Read the model definition and answer for the solid it produces. Units are mm, in the model's axes. A direction names the side the tool comes from. Coordinates: 2 decimals unless noted, no trailing zeros. Order: outer loops, then holes, each group sorted by start corner. A loop starts at its lowest first (then second) coordinate and runs counter-clockwise, first axis right, second up. Notation, with made-up numbers: (-2, 55) - (2, 55) arc R38 ccw to (2, 93) - close; hole circle Ø3 at (87, 69.5). An arc over 180 degrees is marked (long way). Answer as a JSON object with one key per item and string values. Group by question number.
from build123d import *

# Parameters (mm, degrees)
BOSS_EXTRUDE1_DEPTH = 2
BOSS_EXTRUDE2_DEPTH = 2
SKETCH3_R           = 1.2
CUT_EXTRUDE1_DEPTH  = 5
SKETCH4_W           = 6
SKETCH4_H           = 6
CUT_EXTRUDE2_DEPTH  = 5


with BuildPart() as part:
    # Sketch1 → Boss-Extrude1 (new body)
    with BuildSketch(Plane(origin=(0, 0, 0), x_dir=(1, 0, 0), z_dir=(0, 1, 0))):
        with BuildLine():
            Line((-6.5, 2), (6.5, 2))
            ThreePointArc((6.5, 2), (8.5, 0), (6.5, -2))
            Line((6.5, -2), (-6.5, -2))
            ThreePointArc((-6.5, -2), (-8.5, 0), (-6.5, 2))
        make_face()
    extrude(amount=BOSS_EXTRUDE1_DEPTH)

    # Sketch2 → Boss-Extrude2 (add)
    with BuildSketch(Plane.XZ):
        with BuildLine():
            Line((-6.5, 1.15), (6.5, 1.15))
            ThreePointArc((6.5, 1.15), (7.65, 0), (6.5, -1.15))
            Line((6.5, -1.15), (-6.5, -1.15))
            ThreePointArc((-6.5, -1.15), (-7.65, 0), (-6.5, 1.15))
        make_face()
    extrude(amount=BOSS_EXTRUDE2_DEPTH)

    # Sketch3 → Cut-Extrude1 (cut, through all)
    with BuildSketch(Plane.XZ.offset(2)):
        Circle(SKETCH3_R)
    extrude(amount=-CUT_EXTRUDE1_DEPTH, mode=Mode.SUBTRACT)

    # Sketch4 → Cut-Extrude2 (cut, through all)
    with BuildSketch(Plane.XZ.offset(2)):
        with Locations((-7.5, 0)):
            Rectangle(SKETCH4_W, SKETCH4_H)
    extrude(amount=-CUT_EXTRUDE2_DEPTH, mode=Mode.SUBTRACT)


solid = part.part
1. A cutting plane is placed at A-A on x = 0. Write down the section's boundary in (y, z), and give its area (3 significant figures).
2. Given pin 1 (1.6 mm diameter, centred on x = -3.5, y = -1, fed in from +Z); pin 2 (1.6 mm diameter, centred on x = 2, y = -1, fed in from -Z); pin 3 (0.6 mm diameter, centred on x = 3, y = -0.5, fed in from +Z), each flat-ended and moving along its own axis, determine where each tip first touches the part or whether it passes through.
3. A cutting plane is placed at B-B on z = 0. Write down the section's boundary in (x, y), and give its area (3 significant figures).
4. A cutting plane is placed at C-C on y = -0.15. Write down the section's boundary in (x, z), and give its area (3 significant figures).
5. For faces 1 (the flat face through (2.1, 0, -1.4)), 2 (the flat face through (3, -1, 1.15)), 3 (the flat face through (3, -1, -1.15)), 4 (the flat face through (1, 1, 2)), 5 (the flat face through (-3, -2, 0)), determine the directions among +Z, -Z, +X, -X, +Y, -Y from which every point of the face is accessible in a straight line to the end or side of a thin tool.
6. For a pull along X with two mould halves and no side action, classify faces 6 (the cylindrical face through (1.145, -0.028, 0.36)), 7 (the flat face through (1, 1, -2)), 8 (the cylindrical face through (8.5, 1, 0)), 9 (the flat face through (-4.5, 0, 0)) as pulls with the +X half, pulls with the -X half, needs draft (parallel to the pull), parting line crosses it, or undercut.
7. Straight lines are drawn through the part: L1, parallel to X at y = 0.1, z = 0; L2, parallel to X at y = -0.9, z = 0; L3, parallel to Z at x = 0, y = 0.2. For each, find the intervals that lie inside material, in ascending order.
8. A cutting plane is placed at D-D on x = 3.75. Write down the section's boundary in (y, z), and give its area (3 significant figures).
Derived:
{
 "1": {"outline": "(0, -2) - (2, -2) - (2, -1.2) - (0, -1.2) - close; (0, 1.2) - (2, 1.2) - (2, 2) - (0, 2) - close", "area": "3.20 mm2"},
 "2": {"pin 1": "stops at z = 1.15", "pin 2": "stops at z = -1.15", "pin 3": "stops at z = 1.15"},
 "3": {"outline": "(-4.5, -2) - (-1.2, -2) - (-1.2, 2) - (-4.5, 2) - close; (1.2, -2) - (7.65, -2) - (7.65, 0) - (8.5, 0) - (8.5, 2) - (1.2, 2) - close", "area": "40.7 mm2"},
 "4": {"outline": "(-4.5, -1.15) - (-0.34, -1.15) arc R1.2 cw to (-0.34, 1.15) - (-4.5, 1.15) - close; (0.34, -1.15) - (6.5, -1.15) arc R1.15 ccw to (6.5, 1.15) - (0.34, 1.15) arc R1.2 cw to start", "area": "22.9 mm2"},
 "5": {"face 1": "+X, -Y", "face 2": "+Z, +X, -X, -Y", "face 3": "-Z, +X, -X, -Y", "face 4": "+Z, +X, -X, +Y, -Y", "face 5": "+Z, -Z, +X, -X, -Y"},
 "6": {"face 6": "undercut", "face 7": "needs draft", "face 8": "pulls with the +X half", "face 9": "pulls with the -X half"},
 "7": {"L1": "x = -4.5 to -1.2, 1.2 to 8.5", "L2": "x = -4.5 to -1.2, 1.2 to 7.65", "L3": "z = -2 to -1.2, 1.2 to 2"},
 "8": {"outline": "(-2, -1.15) - (0, -1.15) - (0, -2) - (2, -2) - (2, 2) - (0, 2) - (0, 1.15) - (-2, 1.15) - close", "area": "12.6 mm2"}
}
